The drawing under review shows one solid part. Ordinate dimensions are in mm from its lowest x, y, z. Coordinates: 2 decimals unless noted, no trailing zeros. Order: outer loops, then holes, each group sorted by start corner. A loop starts at its lowest first (then second) coordinate and runs counter-clockwise, first axis right, second up.
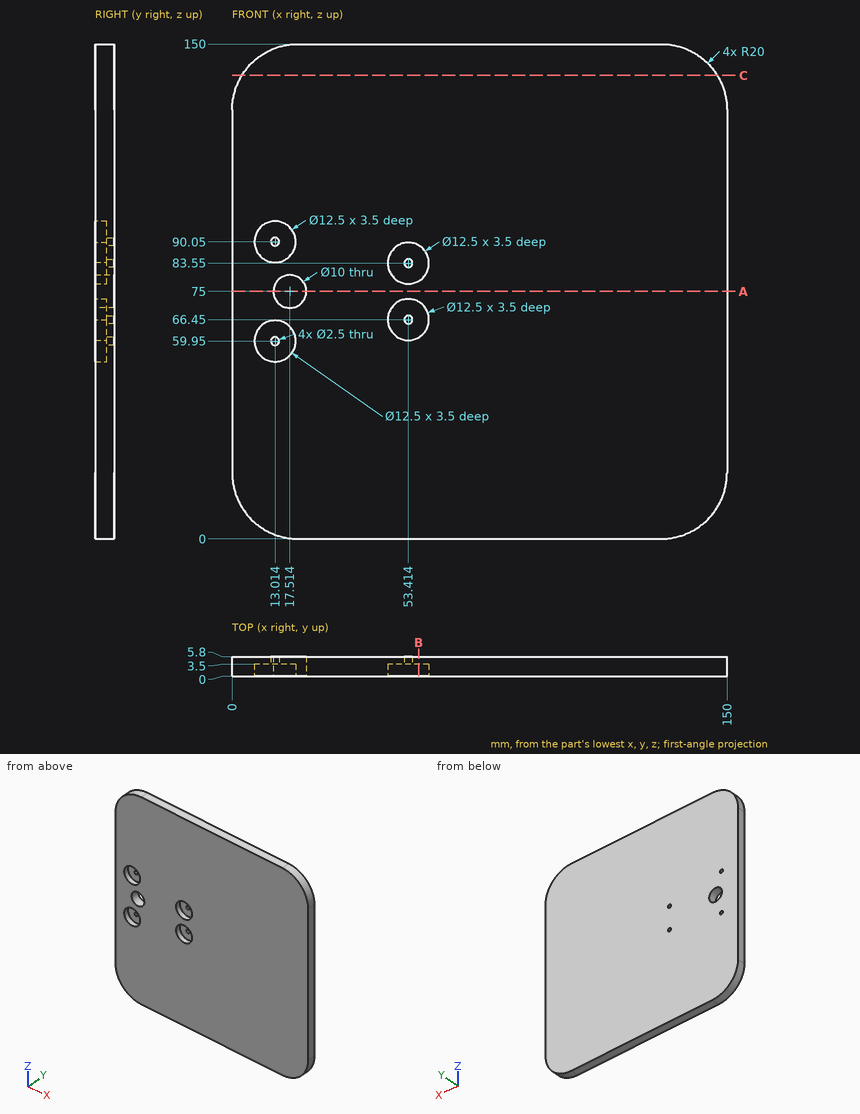
1. To check wall thickness, follow line 1 (X direction, y = 4.9, z = 59.95); line 2 (X direction, y = 1.7, z = 83.55); line 3 (Z direction, x = 18, y = 4.9). State the ranges of each line that lie inside material, in increasing order.
2. Add section B-B (x = 56.5). Give the boundary of the cut face in (y, z) (1 decimal), and give its area (3 significant figures).
3. Add section A-A (z = 75). Give the boundary of the cut face in (x, y), and give its area (3 significant figures).
4. Add section C-C (z = 140.5). Give the boundary of the cut face in (x, y).
5. Insertion check: pin 1 (3 mm diameter, centred on y = 4.5, z = 132.5, fed in from +X) (3 decimals); pin 2 (7.5 mm diameter, centred on x = 53.41, z = 83.55, fed in from -Y); pin 3 (6 mm diameter, centred on x = 17.51, z = 75, fed in from +Y). Each pin has a flat end and moves straight along its axis. Give the tip position at first contact, or say it passes through.
Solution:
1. line 1: x = 0 to 11.76, 14.26 to 150
1. line 2: x = 0 to 47.16, 59.66 to 150
1. line 3: z = 0.1 to 70.02, 79.98 to 149.9
2. outline: (0, 0) - (5.8, 0) - (5.8, 150) - (0, 150) - (0, 89) - (3.5, 89) - (3.5, 78.1) - (0, 78.1) - (0, 71.9) - (3.5, 71.9) - (3.5, 61) - (0, 61) - close
2. area: 794 mm2
3. outline: (0, 0) - (12.51, 0) - (12.51, 5.8) - (0, 5.8) - close; (22.51, 0) - (150, 0) - (150, 5.8) - (22.51, 5.8) - close
3. area: 812 mm2
4. outline: (2.98, 0) - (147.02, 0) - (147.02, 5.8) - (2.98, 5.8) - close
5. pin 1: stops at x = 149.975
5. pin 2: stops at y = 3.5
5. pin 3: passes through
